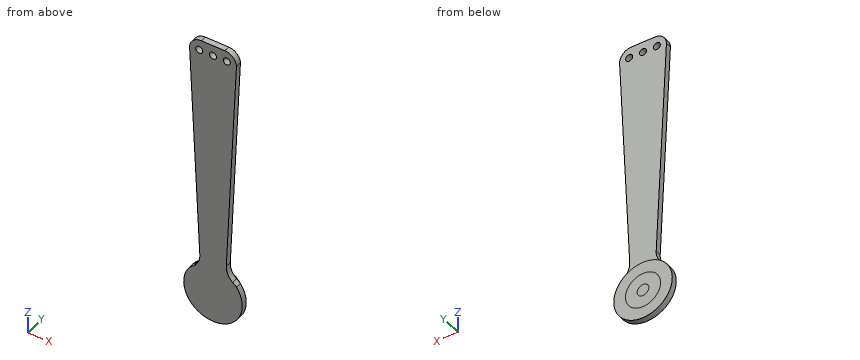
from build123d import *

# Parameters (mm, degrees)
SKETCH2_R           = 25
BOSS_EXTRUDE2_DEPTH = 5
SKETCH3_R           = 15
BOSS_EXTRUDE3_DEPTH = 0.0001
SKETCH4_R           = 5
BOSS_EXTRUDE4_DEPTH = 0.0001
SKETCH20_R          = 3
BOSS_EXTRUDE8_DEPTH = 4.9999
FILLET6_R           = 10
CUT_EXTRUDE4_DEPTH  = 4.9999
FILLET8_R           = 15


with BuildPart() as part:
    # Sketch2 → Boss-Extrude2 (new body)
    with BuildSketch(Plane(origin=(0, 0, 0), x_dir=(1, 0, 0), z_dir=(0, 1, 0))):
        with Locations(Location((0, 0, 0), (0, 0, 270))):
            Circle(SKETCH2_R)
    extrude(amount=BOSS_EXTRUDE2_DEPTH)

    # Sketch3 → Boss-Extrude3 (add)
    with BuildSketch(Plane(origin=(0, 5, 0), x_dir=(1, 0, 0), z_dir=(0, 1, 0))):
        with Locations(Location((0, 0, 0), (0, 0, 270))):
            Circle(SKETCH3_R)
    extrude(amount=BOSS_EXTRUDE3_DEPTH)

    # Sketch4 → Boss-Extrude4 (add)
    with BuildSketch(Plane(origin=(0, 5.0001, 0), x_dir=(1, 0, 0), z_dir=(0, 1, 0))):
        with Locations(Location((0, 0, 0), (0, 0, 270))):
            Circle(SKETCH4_R)
    extrude(amount=BOSS_EXTRUDE4_DEPTH)

    # Sketch20 → Boss-Extrude8 (add)
    with BuildSketch(Plane(origin=(0, 0, 0), x_dir=(1, 0, 0), z_dir=(0, 1, 0))):
        Polygon((20, 0), (20, -224), (-20, -224), (-20, 0), (0, 0), align=None)
        with Locations(Location((-11.77, -215, 0), (0, 0, 270))):
            Circle(SKETCH20_R, mode=Mode.SUBTRACT)
        with Locations(Location((11.77, -215, 0), (0, 0, 270))):
            Circle(SKETCH20_R, mode=Mode.SUBTRACT)
        with Locations(Location((0, -215, 0), (0, 0, 270))):
            Circle(SKETCH20_R, mode=Mode.SUBTRACT)
    extrude(amount=BOSS_EXTRUDE8_DEPTH)

    # Fillet6
    fillet6_edges = [part.edges().sort_by_distance(p)[0] for p in [
        (20, 2.49995, 224),
        (-20, 2.49995, 224),
    ]]
    fillet(fillet6_edges, radius=FILLET6_R)

    # Sketch21 → Cut-Extrude4 (cut)
    with BuildSketch(Plane(origin=(0, 4.9999, 0), x_dir=(1, 0, 0), z_dir=(0, 1, 0))):
        Polygon((20, -214), (11.00508109, -22.44745398), (20, -15), align=None)
        Polygon((-20, -214), (-10.890807236, -22.503117956), (-20, -15), align=None)
    extrude(amount=-CUT_EXTRUDE4_DEPTH, mode=Mode.SUBTRACT)

    # Fillet8
    # the kernel refuses this fillet: 15 mm, written as the material it adds along each edge
    with BuildSketch(Plane(origin=(11.00508109, 4.9999, 22.44745398), x_dir=(0.7702520044264655, 0, -0.6377396409797748), z_dir=(0, -1, 0))) as fillet8_piece_1:
        with BuildLine():
            CenterArc((FILLET8_R * 0.499290509881, FILLET8_R), FILLET8_R, 216.934957366, 53.065042634)
            Line((-FILLET8_R * 0.300027670723, FILLET8_R * 0.399091981951), (0, 0))
            Line((0, 0), (FILLET8_R * 0.499290509881, 0))
        make_face()
    extrude(amount=4.9999)
    with BuildSketch(Plane(origin=(-10.890807236, 4.9999, 22.503117956), x_dir=(-0.04751463426257685, 0, 0.9988705419276782), z_dir=(0, -1, 0))) as fillet8_piece_2:
        with BuildLine():
            CenterArc((FILLET8_R * 0.501260466094, FILLET8_R), FILLET8_R, 216.754404895, 53.245595105)
            Line((-FILLET8_R * 0.299947345081, FILLET8_R * 0.401613800867), (0, 0))
            Line((0, 0), (FILLET8_R * 0.501260466094, 0))
        make_face()
    extrude(amount=4.9999)


solid = part.part
Can you work these out from the model? Positions are in its coordinate system, mm. Round coordinates to 2 decimals unless told otherwise and drop trailing zeros. Order: outer loops, then holes, each group sorted by start corner. A loop starts at its lowest first (then second) coordinate and runs counter-clockwise, first axis right, second up. Notation, with made-up numbers: M 57,67 L 82,67 A20 ccw 82,99 Z; hole C -19,-33.5 d11. An arc over 180 degrees is marked long. Use a Markdown table: item, result.
1) If I drill on line 1 along X through (y, z) = (1.7, 215); line 2 along Z through (x, y) = (-2, 2.85); line 3 along X through (y, z) = (1.5, 130), over which ranges is the centre line in solid material (lowest first)?
Geometry says:
| item | result |
|---|---|
| line 1 | x = -19.95 to -14.77, -8.77 to -3, 3 to 8.77, 14.77 to 19.95 |
| line 2 | z = -24.92 to 212.76, 217.24 to 224 |
| line 3 | x = -16 to 16.06 |
2) I'm going to push flat-ended pins straight in: P1, Ø1.7, axis at x = -18, z = 18.5, coming from the -Y side; P2, Ø5, axis at x = 11.77, z = 215, coming from the +Y side; P3, Ø2, axis at y = 2.5, z = 57, coming from the -X side; P4, Ø1.5, axis at x = -7, y = 3, coming from the -Z side. Where does each tip first touch, or does it pass through?
Geometry says:
| item | result |
|---|---|
| P1 | stops at y = 5 |
| P2 | passes through |
| P3 | stops at x = -12.58 |
| P4 | stops at z = -24.21 |
3) Imagine slicing it at C-C (z = 208.5). List the corners of the cut face in (x, y) for me.
Geometry says:
| item | result |
|---|---|
| outline | M -19.74,0 L 19.74,0 L 19.74,5 L -19.74,5 Z |
4) Imagine slicing it at A-A (y = 3.9). List the corners of the cut face in (x, z) for me, then the cut area to 3 significant figures.
Geometry says:
| item | result |
|---|---|
| outline | M -20,15 A25 ccw long 20,15 L 16.77,17.67 A15 cw 11.36,29.93 L 20,214 A10 ccw 10,224 L -10,224 A10 ccw -20,214 L -11.25,30.01 A15 cw -16.69,17.72 Z; hole C -11.77,215 d6; hole C 0,215 d6; hole C 11.77,215 d6 |
| area | 8,130 mm² |
5) Imagine slicing it at D-D (z = 169). List the corners of the cut face in (x, y) for me.
Geometry says:
| item | result |
|---|---|
| outline | M -17.86,0 L 17.89,0 L 17.89,5 L -17.86,5 Z |
